For this review, take the finished solid that the model builds, in its own axes (mm). A direction names the side the tool comes from. Coordinates: 2 decimals unless noted, no trailing zeros. Loops run counter-clockwise (first coordinate to the right, second up) from the corner with the lowest first, then second, coordinate; pieces in that order, holes last. Notation, with made-up numbers: (75, -26) - (105, -26) arc R22 ccw to (105, 11) - close; hole circle Ø10 at (-3, 51.5). An arc over 180 degrees is marked (long way). One line per item, written item: value. Start each with the question number.
1. Take a section at A-A, the plane x = 0. State the section outline as (y, z) points (3 decimals).
2. Insertion check: pin 1 (7 mm diameter, centred on x = 0, y = 0, fed in from -Z); pin 2 (5 mm diameter, centred on x = 1, y = 0, fed in from +Z). Each pin has a flat end and moves straight along its axis. Give the tip position at first contact, or say it passes through.
3. Take a section at C-C, the plane z = 8. State the section outline as (x, y) points (3 decimals), and give its area (3 significant figures).
4. For faces 5 (the face through (-6.35, 0, 13)), 6 (the face through (-2, 3, 12.7)), list the 3-axis set-ups (+Z, -Z, +X, -X, +Y, -Y) from which the entire face can be reached by the end or side of a thin tool; tool diameter is ignored.
5. To check wall thickness, follow line 1 (Y direction, x = 0, z = 2.5) (3 decimals); line 2 (Z direction, x = -2.5, y = -2.5); line 3 (Y direction, x = 0, z = 19.25). State the ranges of each line that lie inside material, in increasing order. Write a range as from..to.
6. Take a section at D-D, the plane y = 3.5. State the section outline as (x, z) points.
7. The part is to be moulded in two halves that separate along Y. For faces 1 (the face through (-0.86, -3.874, 19.139)), 2 (the face through (6.35, 0, 13)), 3 (the face through (0, 6.35, 13)), 4 (the face through (0, -6.35, 13)), say which applies: released by +Y, released by -Y, zero draft, split by the parting line, or undercut.
```python
from build123d import *

# Parameters (mm, degrees)
SKETCH1_W           = 12.7
SKETCH1_H           = 12.7
BOSS_EXTRUDE1_DEPTH = 25.4
SKETCH2_R           = 3.175
CUT_EXTRUDE1_DEPTH  = 12.7
SKETCH3_R           = 3.96875
CUT_EXTRUDE2_DEPTH  = 12.7


with BuildPart() as part:
    # Sketch1 → Boss-Extrude1 (new body)
    with BuildSketch(Plane.XY):
        Rectangle(SKETCH1_W, SKETCH1_H)
    extrude(amount=BOSS_EXTRUDE1_DEPTH)

    # Sketch2 → Cut-Extrude1 (cut)
    with BuildSketch(Plane(origin=(0, 0, 0), x_dir=(-1, 0, 0), z_dir=(0, 0, -1))):
        Circle(SKETCH2_R)
    extrude(amount=-CUT_EXTRUDE1_DEPTH, mode=Mode.SUBTRACT)

    # Sketch3 → Cut-Extrude2 (cut)
    with BuildSketch(Plane.XY.offset(25.4)):
        Circle(SKETCH3_R)
    extrude(amount=-CUT_EXTRUDE2_DEPTH, mode=Mode.SUBTRACT)


solid = part.part
```
Solutions:
1. outline: (-6.35, 0) - (-3.175, 0) - (-3.175, 12.7) - (-3.969, 12.7) - (-3.969, 25.4) - (-6.35, 25.4) - close; (3.175, 0) - (6.35, 0) - (6.35, 25.4) - (3.969, 25.4) - (3.969, 12.7) - (3.175, 12.7) - close
2. pin 1: z = 0
2. pin 2: z = 12.7
3. outline: (-6.35, -6.35) - (6.35, -6.35) - (6.35, 6.35) - (-6.35, 6.35) - close; hole circle Ø6.35 at (0, 0)
3. area: 130 mm2
4. face 5: +Z, -Z, -X, +Y, -Y
4. face 6: +Z
5. line 1: -6.35..-3.175, 3.175..6.35
5. line 2: 0..12.7
5. line 3: -6.35..-3.97, 3.97..6.35
6. outline: (-6.35, 0) - (6.35, 0) - (6.35, 25.4) - (1.87, 25.4) - (1.87, 12.7) - (-1.87, 12.7) - (-1.87, 25.4) - (-6.35, 25.4) - close
7. face 1: undercut
7. face 2: zero draft
7. face 3: released by +Y
7. face 4: released by -Y
